from build123d import *

# Parameters (mm, degrees)
SKETCH1_R                  = 19.05
BOSS_EXTRUDE1_DEPTH        = 6.35
SKETCH2_R                  = 10.16
BOSS_EXTRUDE2_DEPTH        = 19.05
F_0_257_DIAMETER_HOLE1_D   = 6.5278
F_10_24_TAPPED_HOLE3_D     = 3.9878
F_10_24_TAPPED_HOLE3_DEPTH = 10.159
F_10_24_TAPPED_HOLE3_TIP   = 1.198055988
H_0_266_DIAMETER_HOLE1_D   = 6.7564


with BuildPart() as part:
    # Sketch1 → Boss-Extrude1 (new body)
    with BuildSketch(Plane.XY):
        Circle(SKETCH1_R)
    extrude(amount=BOSS_EXTRUDE1_DEPTH)

    # Sketch2 → Boss-Extrude2 (add)
    with BuildSketch(Plane(origin=(0, 0, 0), x_dir=(-1, 0, 0), z_dir=(0, 0, -1))):
        Circle(SKETCH2_R)
    extrude(amount=-BOSS_EXTRUDE2_DEPTH)

    # F (0.257) Diameter Hole1 (through all)
    with Locations(Plane.XY.offset(19.05)):
        with Locations((0, 0)):
            Hole(F_0_257_DIAMETER_HOLE1_D / 2)

    # #10-24 Tapped Hole3
    with Locations(Plane(origin=(0, 10.16, 12.7), x_dir=(0, 0, 1), z_dir=(0, 1, 0))):
        with Locations((0, 0)):
            Hole(F_10_24_TAPPED_HOLE3_D / 2, depth=F_10_24_TAPPED_HOLE3_DEPTH)
            with Locations((0, 0, -(F_10_24_TAPPED_HOLE3_DEPTH + F_10_24_TAPPED_HOLE3_TIP / 2))):  # 118° drill point
                Cone(0, F_10_24_TAPPED_HOLE3_D / 2, F_10_24_TAPPED_HOLE3_TIP, mode=Mode.SUBTRACT)

    # H (0.266) Diameter Hole1 (through all)
    with Locations(Plane.XY.offset(6.35)):
        with Locations((-14.605, 0), (14.605, 0)):
            Hole(H_0_266_DIAMETER_HOLE1_D / 2)


solid = part.part
The listing builds one solid part. Answer for the finished solid, in the listing's coordinates (mm). A direction names the side the tool comes from. Round coordinates to 2 decimals unless told otherwise and drop trailing zeros. Write each loop counter-clockwise with the first axis right and the second up, starting at its lowest first coordinate (ties: lowest second). Pieces come first, ordered by that corner, then holes. Notation, with made-up numbers: (36.5, 7.5) - (54.5, 7.5) arc R8 ccw to (54.5, 22.5) - close; hole circle Ø4 at (8, 24). An arc over 180 degrees is marked (long way). Use a Markdown table: item, result. Add a question column.
1. A tool of negligible diameter and unlimited length cuts with its end or side. For faces 4 (the face through (-4, 0, 0)), 5 (the face through (0.6, 6.3, 10.8)), from which of +Z, -Z, +X, -X, +Y, -Y can it reach the whole face along a straight path? Write none if from no direction.
2. For a pull along X with two mould halves and no side action, classify faces 1 (the face through (11.484, -1.294, 3.131)), 2 (the face through (2.2, -9.92, 12.61)), 3 (the face through (8, -8, 6.35)) as +X half, -X half, draft (parallel to the pull), parting line (faces both ways), or undercut.
3. Consider line 1 (Y direction, x = 0, z = 2.75); line 2 (Z direction, x = -4, y = 11); line 3 (Y direction, x = -17, z = 6). Determine where each line is inside the solid, lowest interval first.
4. The part is cut by section A-A (y = 0). Write down the section's boundary in (x, z), and give its area (3 significant figures).
5. The part is cut by section D-D (y = 4.5). Write down the section's boundary in (x, z).
6. The part is cut by section C-C (x = -13). Write down the section's boundary in (y, z), and give its area (3 significant figures).
7. The part is cut by section B-B (x = 0). Write down the section's boundary in (y, z).
8. Flat-ended cylindrical pins translate along their axes: P1, Ø4, axis at x = -1.5, z = 4, coming from the -Y side; P2, Ø3, axis at y = 4, z = 13.5, coming from the +X side; P3, Ø1.5, axis at x = 1, y = 1.5, coming from the +Z side; P4, Ø2, axis at x = 0.5, z = 16, coming from the +Y side. Find the tip coordinate at first contact, or state that the pin passes through.
Reported:
| question | item | result |
|---|---|---|
| 1 | face 4 | -Z, +X, -X, +Y, -Y |
| 1 | face 5 | +Y |
| 2 | face 1 | undercut |
| 2 | face 2 | parting line |
| 2 | face 3 | draft |
| 3 | line 1 | -19.05 to -3.26, 3.26 to 19.05 |
| 3 | line 2 | 0 to 6.35 |
| 3 | line 3 | -8.6 to -2.38, 2.38 to 8.6 |
| 4 | outline | (-19.05, 0) - (-17.98, 0) - (-17.98, 6.35) - (-19.05, 6.35) - close; (-11.23, 0) - (-3.26, 0) - (-3.26, 19.05) - (-10.16, 19.05) - (-10.16, 6.35) - (-11.23, 6.35) - close; (3.26, 0) - (11.23, 0) - (11.23, 6.35) - (10.16, 6.35) - (10.16, 19.05) - (3.26, 19.05) - close; (17.98, 0) - (19.05, 0) - (19.05, 6.35) - (17.98, 6.35) - close |
| 4 | area | 290 mm^2 |
| 5 | outline | (-18.51, 0) - (18.51, 0) - (18.51, 6.35) - (9.11, 6.35) - (9.11, 19.05) - (-9.11, 19.05) - (-9.11, 6.35) - (-18.51, 6.35) - close; hole circle Ø3.99 at (0, 12.7) |
| 6 | outline | (-13.92, 0) - (-2.97, 0) - (-2.97, 6.35) - (-13.92, 6.35) - close; (2.97, 0) - (13.92, 0) - (13.92, 6.35) - (2.97, 6.35) - close |
| 6 | area | 139 mm^2 |
| 7 | outline | (-19.05, 0) - (-3.26, 0) - (-3.26, 19.05) - (-10.16, 19.05) - (-10.16, 6.35) - (-19.05, 6.35) - close; (3.26, 0) - (19.05, 0) - (19.05, 6.35) - (10.16, 6.35) - (10.16, 10.71) - (3.26, 10.71) - close; (3.26, 14.69) - (10.16, 14.69) - (10.16, 19.05) - (3.26, 19.05) - close |
| 8 | P1 | y = -19.05 |
| 8 | P2 | x = 9.85 |
| 8 | P3 | through |
| 8 | P4 | y = 10.16 |
